```python
from build123d import *

# Parameters (mm, degrees)
SKETCH1_W                                           = 343
SKETCH1_H                                           = 200
EXTRUDE1_DEPTH                                      = 4
CSK_FOR_M3_COUNTERSUNK_FLAT_HEAD_SCREW1_D           = 3.4
CSK_FOR_M3_COUNTERSUNK_FLAT_HEAD_SCREW1_CSINK_D     = 6.3
CSK_FOR_M3_COUNTERSUNK_FLAT_HEAD_SCREW1_CSINK_ANGLE = 90
CSK_FOR_M4_COUNTERSUNK_FLAT_HEAD_SCR_2_COUNT        = 2
CSK_FOR_M4_COUNTERSUNK_FLAT_HEAD_SCR_2_PITCH        = 331
LPATTERN1_COUNT                                     = 4
LPATTERN1_PITCH                                     = 38.4


with BuildPart() as part:
    # Sketch1 → Extrude1 (new body)
    with BuildSketch(Plane.XY):
        with Locations((171.5, 100)):
            Rectangle(SKETCH1_W, SKETCH1_H)
    extrude(amount=EXTRUDE1_DEPTH)

    # CSK for M3 Countersunk Flat Head Screw1 (through all)
    with Locations(Plane(origin=(6, 196, 4), x_dir=(1, 0, 0), z_dir=(0, 0, 1))):
        with Locations((0, 0), (0, -192), (331, -192), (331, 0)):
            CounterSinkHole(CSK_FOR_M3_COUNTERSUNK_FLAT_HEAD_SCREW1_D / 2, CSK_FOR_M3_COUNTERSUNK_FLAT_HEAD_SCREW1_CSINK_D / 2, counter_sink_angle=CSK_FOR_M3_COUNTERSUNK_FLAT_HEAD_SCREW1_CSINK_ANGLE)

    # Sketch4 → CSK for M4 Countersunk Flat Head Screw1 (revolve, cut)
    with BuildSketch(Plane(origin=(6, 42.4, 4), x_dir=(0, -1, 0), z_dir=(1, 0, 0))):
        Polygon((0, 0), (0, 4), (2.25, 4), (2.25, 2.45), (4.7, 0), align=None)
    csk_for_m4_countersunk_flat_head_screw1 = revolve(axis=Axis((6, 42.4, 10.35), (0, 0, -1)), mode=Mode.SUBTRACT)

    # CSK for M4 Countersunk Flat Head Scr 2: CSK for M4 Countersunk Flat Head Screw1 ×2
    with Locations(*[(i * CSK_FOR_M4_COUNTERSUNK_FLAT_HEAD_SCR_2_PITCH, 0, 0) for i in range(1, CSK_FOR_M4_COUNTERSUNK_FLAT_HEAD_SCR_2_COUNT)]):
        add(csk_for_m4_countersunk_flat_head_screw1, mode=Mode.SUBTRACT)

    # LPattern1: CSK for M4 Countersunk Flat Head Screw1 ×4
    with Locations(*[(0, i * LPATTERN1_PITCH, 0) for i in range(1, LPATTERN1_COUNT)]):
        add(csk_for_m4_countersunk_flat_head_screw1, mode=Mode.SUBTRACT)

    # LPattern1 copy 1 sketch → LPattern1 copy 1 (revolve, cut)
    with BuildSketch(Plane(origin=(337, 80.8, 4), x_dir=(0, -1, 0), z_dir=(1, 0, 0))):
        Polygon((0, 0), (0, 4), (2.25, 4), (2.25, 2.45), (4.7, 0), align=None)
    revolve(axis=Axis((337, 80.8, 10.35), (0, 0, -1)), mode=Mode.SUBTRACT)

    # LPattern1 copy 2 sketch → LPattern1 copy 2 (revolve, cut)
    with BuildSketch(Plane(origin=(337, 119.2, 4), x_dir=(0, -1, 0), z_dir=(1, 0, 0))):
        Polygon((0, 0), (0, 4), (2.25, 4), (2.25, 2.45), (4.7, 0), align=None)
    revolve(axis=Axis((337, 119.2, 10.35), (0, 0, -1)), mode=Mode.SUBTRACT)

    # LPattern1 copy 3 sketch → LPattern1 copy 3 (revolve, cut)
    with BuildSketch(Plane(origin=(337, 157.6, 4), x_dir=(0, -1, 0), z_dir=(1, 0, 0))):
        Polygon((0, 0), (0, 4), (2.25, 4), (2.25, 2.45), (4.7, 0), align=None)
    revolve(axis=Axis((337, 157.6, 10.35), (0, 0, -1)), mode=Mode.SUBTRACT)


solid = part.part
```
Could you check a few things on this model? Use its own coordinates, in mm. Coordinates: 2 decimals unless noted, no trailing zeros.
1) Will these pins go through, and if not, where does the flat tip stop? pin 1 Ø3 at (x, y) = (6, 196) entering from +Z; pin 2 Ø6 at (x, y) = (337, 157.6) entering from +Z.
Reported:
pin 1: passes through
pin 2: stops at z = 2.3
2) Thinking about a two-plate mould opening in Y: for faces 1 (the face through (334.62, 81.11, 1.7)), 2 (the face through (169, 101, 4)), 3 (the face through (334.62, 157.91, 1.7)), which applies, released by +Y, released by -Y, zero draft, split by the parting line, or undercut?
Reported:
face 1: undercut
face 2: zero draft
face 3: undercut
3) Please list where these lines run through material, in increasing order: line 1 along X through (y, z) = (119.2, 1.1); line 2 along X through (y, z) = (120.5, 1.6).
Reported:
line 1: x = 0 to 3.75, 8.25 to 334.75, 339.25 to 343
line 2: x = 0 to 4.1, 7.9 to 335.1, 338.9 to 343
